Input: dimensioned drawing with shaded views. Units: mm. Origin: part minimum x, y, z. Give positions to 0.01 mm unless a question says otherwise; leave off trailing zeros. Order: outer loops, then holes, each group sorted by start corner. A loop starts at its lowest first (then second) coordinate and runs counter-clockwise, first axis right, second up.
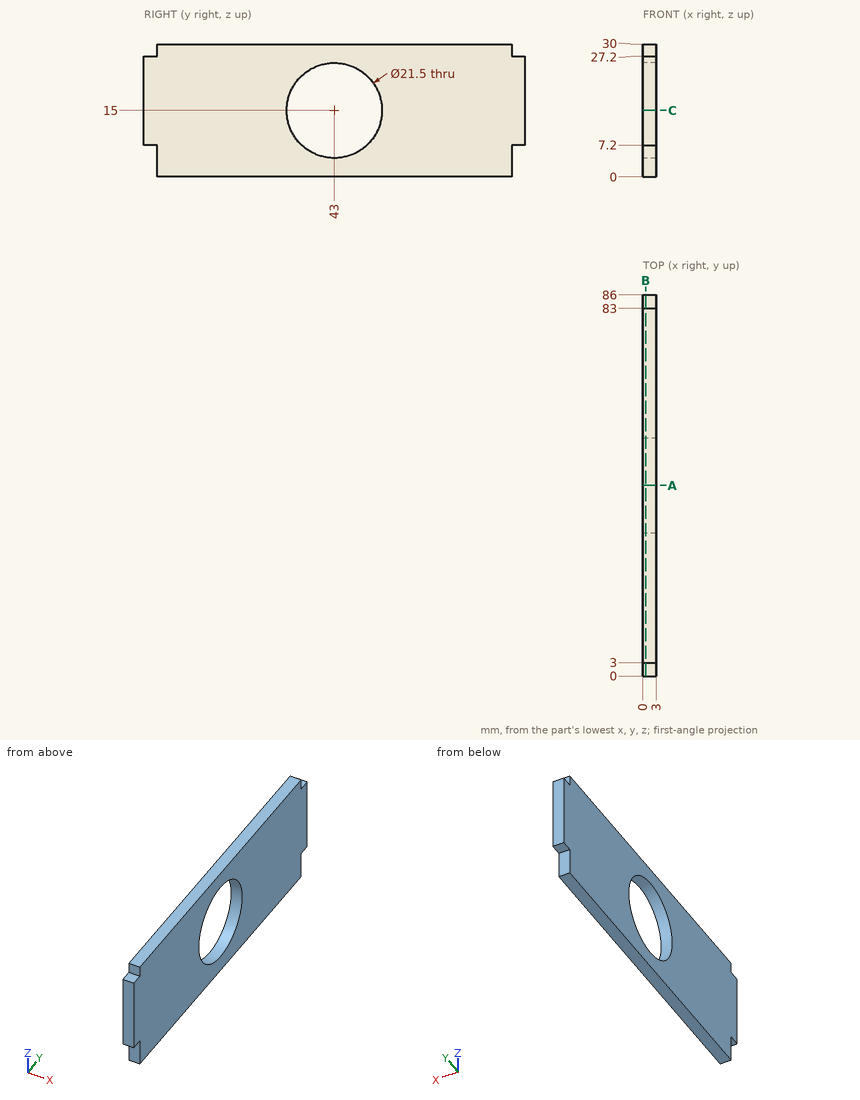
1) Section query A-A, the plane y = 43. Return the cut outline in (x, z), and give its area (3 significant figures).
Report:
outline: (0, 0) - (3, 0) - (3, 4.25) - (0, 4.25) - close; (0, 25.75) - (3, 25.75) - (3, 30) - (0, 30) - close
area: 25.5 mm2
2) Pin query (flat end, axial travel): pin 1 (6 mm diameter, centred on y = 72, z = 5.5, fed in from -X); pin 2 (0.9 mm diameter, centred on x = 1, y = 1.5, fed in from +Z); pin 3 (1.5 mm diameter, centred on x = 2, z = 3.5, fed in from +Y); pin 4 (1.5 mm diameter, centred on x = 1, z = 4.5, fed in from -Y). Return the tip coordinate at first contact, or that it passes through.
Report:
pin 1: stops at x = 0
pin 2: stops at z = 27.2
pin 3: stops at y = 83
pin 4: stops at y = 3
3) Material intervals for L1, parallel to Z at x = 2.45, y = 43; L2, parallel to Y at x = 0.55, z = 15.5; L3, parallel to Z at x = 1.1, y = 48, sorted ascending.
Report:
L1: z = 0 to 4.25, 25.75 to 30
L2: y = 0 to 32.26, 53.74 to 86
L3: z = 0 to 5.48, 24.52 to 30
4) Section query B-B, the plane x = 0.6. Return the cut outline in (y, z).
Report:
outline: (0, 7.2) - (3, 7.2) - (3, 0) - (83, 0) - (83, 7.2) - (86, 7.2) - (86, 27.2) - (83, 27.2) - (83, 30) - (3, 30) - (3, 27.2) - (0, 27.2) - close; hole circle Ø21.5 at (43, 15)
5) Section query C-C, the plane z = 15. Return the cut outline in (x, y), and give its area (4 significant figures).
Report:
outline: (0, 0) - (3, 0) - (3, 32.25) - (0, 32.25) - close; (0, 53.75) - (3, 53.75) - (3, 86) - (0, 86) - close
area: 193.5 mm2
